from build123d import *

# Parameters (mm, degrees)
F0_R     = 25
F1_DEPTH = 3
F2_R     = 25
F2_R_2   = 21
F3_DEPTH = 50
F4_R     = 1.99999
F5_R     = 2


# Not quite as in the source:
# - a fillet or chamfer is up to 0.001 mm smaller than in the source, because OpenCascade refuses the exact size


with BuildPart() as f1:
    # F0 (on Top) → F1 (new body)
    with BuildSketch(Plane.XY):
        Circle(F0_R)
    extrude(amount=F1_DEPTH)

    # F2 (on face) → F3 (join)
    with BuildSketch(Plane.XY.offset(3)):
        Circle(F2_R)
        Circle(F2_R_2, mode=Mode.SUBTRACT)
    extrude(amount=F3_DEPTH)

    # F4 (radius 2 in the source; OpenCascade refuses exactly that, so slightly less here)
    f4_edges = [f1.edges().sort_by_distance(p)[0] for p in [
        (-25, 0, 53),
        (-21, 0, 53),
        (-21, 0, 3),
    ]]
    fillet(f4_edges, radius=F4_R)

    # F5
    f5_edges = [f1.edges().sort_by_distance(p)[0] for p in [
        (-25, 0, 0),
    ]]
    fillet(f5_edges, radius=F5_R)


solid = f1.part
Read the model definition and answer for the solid it produces. Units are mm, in the model's axes. Round coordinates to 2 decimals unless told otherwise and drop trailing zeros. Write each loop counter-clockwise with the first axis right and the second up, starting at its lowest first coordinate (ties: lowest second). Pieces come first, ordered by that corner, then holes. Notation, with made-up numbers: (-22.75, -38.5) - (32.25, -38.5) arc R27 cw to (32.25, -11.5) - close; hole circle Ø11 at (15, 68). An arc over 180 degrees is marked (long way). One line per question, with ' | ' between items. Start each with the question number.
1. For a pull along X with two mould halves and no side action, classify faces 1 (the face through (0, 0, 0)), 2 (the face through (0, 0, 3)), 3 (the face through (23.846, 7.509, 26.157)), 4 (the face through (20.03, 6.31, 27.68)) as +X half, -X half, draft (parallel to the pull), parting line (faces both ways), or undercut.
2. Find the intervals of material crossed by probe 1 along X at (y, z) = (0.5, 38) (3 decimals); probe 2 along Y at (x, z) = (0, 40); probe 3 along Z at (x, y) = (10, -9), in increasing order. Write a range as [from, to].
3. Each of these flat-tipped pins is pushed along its axis until it touches: pin 1 (11.5 mm diameter, centred on x = 5, y = 0.5, fed in from +Z); pin 2 (8 mm diameter, centred on x = 13.5, y = -12, fed in from +Z); pin 3 (12 mm diameter, centred on x = -14, z = 10, fed in from -Y). Where does it stop, or does it pass through?
4. Section C-C (z = 43) is taken. Determine the outline of the cut face in (x, y).
Filled in:
1) face 1: draft | face 2: undercut | face 3: parting line | face 4: undercut
2) probe 1: [-24.995, -20.994], [20.994, 24.995] | probe 2: [-25, -21], [21, 25] | probe 3: [0, 3]
3) pin 1: z = 3 | pin 2: z = 52.77 | pin 3: y = -23.69
4) outline: circle Ø50 at (0, 0); hole circle Ø42 at (0, 0)
